Read the model definition and answer for the solid it produces. Units are mm, in the model's axes. Coordinates: 2 decimals unless noted, no trailing zeros. Write each loop counter-clockwise with the first axis right and the second up, starting at its lowest first coordinate (ties: lowest second). Pieces come first, ordered by that corner, then holes. Notation, with made-up numbers: (49.25, -40) - (107.25, -40) arc R20 ccw to (107.25, -21) - close; hole circle Ø11 at (-31.5, -33). An arc over 180 degrees is marked (long way). Use a Markdown table: item, result.
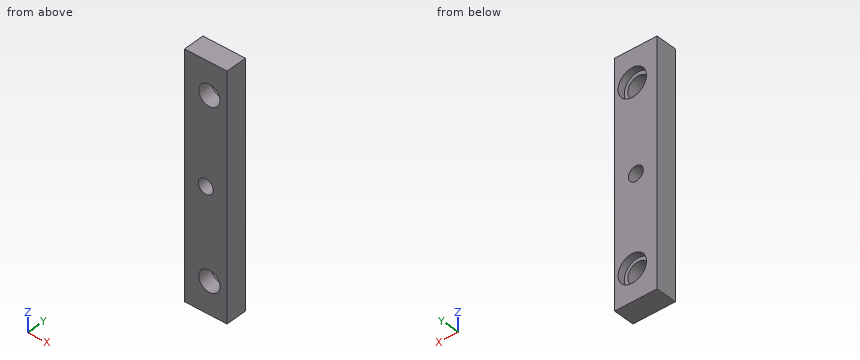
from build123d import *

# Parameters (mm, degrees)
SKETCH1_W             = 12
SKETCH1_H             = 6
BOSS_EXTRUDE1_DEPTH   = 60
SKETCH2_R             = 3
CUT_EXTRUDE1_DEPTH    = 7
SKETCH3_R             = 4
CUT_EXTRUDE2_DEPTH    = 2
SKETCH4_W             = 12
SKETCH4_H             = 6
BOSS_EXTRUDE2_DEPTH   = 4
SKETCH5_W             = 12
SKETCH5_H             = 6
BOSS_EXTRUDE3_DEPTH   = 4
M5_TAPPED_HOLE1_D     = 4.2
M5_TAPPED_HOLE1_DEPTH = 52
M5_TAPPED_HOLE1_TIP   = 1.2618073


with BuildPart() as part:
    # Sketch1 → Boss-Extrude1 (new body)
    with BuildSketch(Plane.XY):
        Rectangle(SKETCH1_W, SKETCH1_H)
    extrude(amount=BOSS_EXTRUDE1_DEPTH)

    # Sketch2 → Cut-Extrude1 (cut, through all)
    with BuildSketch(Plane(origin=(0, 3, 0), x_dir=(1, 0, 0), z_dir=(0, 1, 0))):
        with Locations((1, -5)):
            Circle(SKETCH2_R)
        with Locations((1, -55)):
            Circle(SKETCH2_R)
    extrude(amount=-CUT_EXTRUDE1_DEPTH, mode=Mode.SUBTRACT)

    # Sketch3 → Cut-Extrude2 (cut)
    with BuildSketch(Plane(origin=(0, 3, 0), x_dir=(1, 0, 0), z_dir=(0, 1, 0))):
        with Locations((1, -5)):
            Circle(SKETCH3_R)
        with Locations((1, -55)):
            Circle(SKETCH3_R)
    extrude(amount=-CUT_EXTRUDE2_DEPTH, mode=Mode.SUBTRACT)

    # Sketch4 → Boss-Extrude2 (add)
    with BuildSketch(Plane(origin=(0, 0, 0), x_dir=(-1, 0, 0), z_dir=(0, 0, -1))):
        Rectangle(SKETCH4_W, SKETCH4_H)
    extrude(amount=BOSS_EXTRUDE2_DEPTH)

    # Sketch5 → Boss-Extrude3 (add)
    with BuildSketch(Plane.XY.offset(60)):
        Rectangle(SKETCH5_W, SKETCH5_H)
    extrude(amount=BOSS_EXTRUDE3_DEPTH)

    # M5 Tapped Hole1
    with Locations(Plane(origin=(0, 3, 0), x_dir=(-1, 0, 0), z_dir=(0, 1, 0))):
        with Locations((0, 30)):
            Hole(M5_TAPPED_HOLE1_D / 2, depth=M5_TAPPED_HOLE1_DEPTH)
            with Locations((0, 0, -(M5_TAPPED_HOLE1_DEPTH + M5_TAPPED_HOLE1_TIP / 2))):  # 118° drill point
                Cone(0, M5_TAPPED_HOLE1_D / 2, M5_TAPPED_HOLE1_TIP, mode=Mode.SUBTRACT)


solid = part.part
(1) A cutting plane is placed at A-A, the plane y = -2.1. Write down the section's boundary in (x, z), and give its area (3 significant figures).
Report:
| item | result |
|---|---|
| outline | (-6, -4) - (6, -4) - (6, 64) - (-6, 64) - close; hole circle Ø4.2 at (0, 30); hole circle Ø6 at (1, 5); hole circle Ø6 at (1, 55) |
| area | 746 mm² |
(2) A cutting plane is placed at D-D, the plane z = 30. Write down the section's boundary in (x, y).
Report:
| item | result |
|---|---|
| outline | (-6, -3) - (-2.1, -3) - (-2.1, 3) - (-6, 3) - close; (2.1, -3) - (6, -3) - (6, 3) - (2.1, 3) - close |
(3) Straight lines are drawn through the part: L1, parallel to Z at x = 1, y = 0; L2, parallel to Z at x = -1.5, y = 1.4; L3, parallel to Z at x = 2.75, y = -1.5. For each, find the intervals that lie inside material, in ascending order.
Report:
| item | result |
|---|---|
| L1 | z = -4 to 2, 8 to 28.15, 31.85 to 52, 58 to 64 |
| L2 | z = -4 to 1.88, 8.12 to 28.53, 31.47 to 51.88, 58.12 to 64 |
| L3 | z = -4 to 2.56, 7.44 to 52.56, 57.44 to 64 |
(4) A cutting plane is placed at C-C, the plane x = 0. Write down the section's boundary in (y, z).
Report:
| item | result |
|---|---|
| outline | (-3, -4) - (3, -4) - (3, 1.13) - (1, 1.13) - (1, 2.17) - (-3, 2.17) - close; (-3, 7.83) - (1, 7.83) - (1, 8.87) - (3, 8.87) - (3, 27.9) - (-3, 27.9) - close; (-3, 32.1) - (3, 32.1) - (3, 51.13) - (1, 51.13) - (1, 52.17) - (-3, 52.17) - close; (-3, 57.83) - (1, 57.83) - (1, 58.87) - (3, 58.87) - (3, 64) - (-3, 64) - close |
(5) A cutting plane is placed at B-B, the plane z = 5. Write down the section's boundary in (x, y), and give its area (3 significant figures).
Report:
| item | result |
|---|---|
| outline | (-6, -3) - (-2, -3) - (-2, 1) - (-3, 1) - (-3, 3) - (-6, 3) - close; (4, -3) - (6, -3) - (6, 3) - (5, 3) - (5, 1) - (4, 1) - close |
| area | 32.0 mm² |
